Source: CAD feature listing. Evaluate the final solid. Frame: model axes, mm. A direction names the side the tool comes from. Give positions to 0.01 mm unless a question says otherwise; leave off trailing zeros. Order: outer loops, then holes, each group sorted by start corner. A loop starts at its lowest first (then second) coordinate and runs counter-clockwise, first axis right, second up. Notation, with made-up numbers: (85.5, 23.25) - (142.5, 23.25) arc R23 cw to (142.5, 56.25) - close; hole circle Ø5 at (79, 28.5). An arc over 180 degrees is marked (long way). Use CSV: the item, a comma, the result in double quotes.
```python
from build123d import *

# Parameters (mm, degrees)
SKETCH1_W                       = 88.9
SKETCH1_H                       = 107.95
EXTRUDE1_DEPTH                  = 75
SKETCH2_R                       = 14.2875
EXTRUDE2_DEPTH                  = 203.2
M6_TAPPED_HOLE1_D               = 5
M6_TAPPED_HOLE1_DEPTH           = 27.9908
M6_TAPPED_HOLE1_TIP             = 1.502151548
SKETCH6_R                       = 15.875
EXTRUDE4_DEPTH                  = 38.354
SKETCH7_W                       = 88.9
SKETCH7_H                       = 44.45
EXTRUDE5_DEPTH                  = 25
SKETCH8_W                       = 4.2125
SKETCH8_H                       = 107.95
EXTRUDE6_DEPTH                  = 103.538300771
CBORE_FOR_M20_SHCS1_D           = 22
CBORE_FOR_M20_SHCS1_CBORE_D     = 33
CBORE_FOR_M20_SHCS1_CBORE_DEPTH = 20
CHAMFER1_SIZE                   = 1


with BuildPart() as part:
    # Sketch1 → Extrude1 (new body)
    with BuildSketch(Plane(origin=(0, 0, 0), x_dir=(1, 0, 0), z_dir=(0, 1, 0))):
        Rectangle(SKETCH1_W, SKETCH1_H)
    extrude(amount=EXTRUDE1_DEPTH)

    # Sketch2 → Extrude2 (cut)
    with BuildSketch(Plane(origin=(0, 75, 0), x_dir=(1, 0, 0), z_dir=(0, 1, 0))):
        with Locations(Location((-4.7625, 0, 0), (0, 0, 270))):
            Circle(SKETCH2_R)
    extrude(amount=-EXTRUDE2_DEPTH, mode=Mode.SUBTRACT)

    # M6 Tapped Hole1
    with Locations(Plane.XZ):
        with Locations((-22.9235, 34.925), (13.3985, 34.925), (-22.9235, -34.925), (13.3985, -34.925)):
            Hole(M6_TAPPED_HOLE1_D / 2, depth=M6_TAPPED_HOLE1_DEPTH)
            with Locations((0, 0, -(M6_TAPPED_HOLE1_DEPTH + M6_TAPPED_HOLE1_TIP / 2))):  # 118° drill point
                Cone(0, M6_TAPPED_HOLE1_D / 2, M6_TAPPED_HOLE1_TIP, mode=Mode.SUBTRACT)

    # Sketch6 → Extrude4 (cut)
    with BuildSketch(Plane(origin=(0, 75, 0), x_dir=(1, 0, 0), z_dir=(0, 1, 0))):
        with Locations(Location((-4.7625, 0, 0), (0, 0, 270))):
            Circle(SKETCH6_R)
    extrude(amount=-EXTRUDE4_DEPTH, mode=Mode.SUBTRACT)

    # Sketch7 → Extrude5 (cut)
    with BuildSketch(Plane.XZ):
        Rectangle(SKETCH7_W, SKETCH7_H)
    extrude(amount=-EXTRUDE5_DEPTH, mode=Mode.SUBTRACT)

    # Sketch8 → Extrude6 (cut, through all)
    with BuildSketch(Plane(origin=(0, 75, 0), x_dir=(1, 0, 0), z_dir=(0, 1, 0))):
        with Locations((42.34375, 0)):
            Rectangle(SKETCH8_W, SKETCH8_H)
    extrude(amount=-EXTRUDE6_DEPTH, mode=Mode.SUBTRACT)

    # CBORE for M20 SHCS1 (through all)
    with Locations(Plane.ZY.offset(44.45)):
        with Locations((32.5, 50), (-32.5, 50)):
            CounterBoreHole(CBORE_FOR_M20_SHCS1_D / 2, CBORE_FOR_M20_SHCS1_CBORE_D / 2, CBORE_FOR_M20_SHCS1_CBORE_DEPTH)

    # Chamfer1
    chamfer1_edges = [part.edges().sort_by_distance(p)[0] for p in [
        (-4.7625, 75, -15.875),
    ]]
    chamfer(chamfer1_edges, length=CHAMFER1_SIZE)


solid = part.part
```
Item 1: Mould query, pull axis Z, two halves, no side actions, for faces 6 (the flat face through (-3, 37, -53.975)), 7 (the cylindrical face through (-25.233, 14.191, 33.967)), 8 (the flat face through (-3, 0, 38)). Classes: released by +Z, released by -Z, zero draft, split by the parting line, or undercut.
Filled in:
face 6,"released by -Z"
face 7,"undercut"
face 8,"zero draft"
Item 2: Material intervals for line 1 (Y direction, x = -30.5, z = 32.5); line 2 (Z direction, x = 10.5, y = 3) (3 decimals); line 3 (Z direction, x = -24.5, y = 36) (3 decimals), sorted ascending. Write a range as from..to.
Filled in:
line 1,"y = 0..33.5, 66.5..75"
line 2,"z = -53.975..-22.225, 22.225..53.975"
line 3,"z = -53.975..-41.232, -23.768..23.768, 41.232..53.975"
Item 3: Set-up query: faces 1 (the cylindrical face through (-34.59, 33.892, -36.077)), 2 (the flat face through (-44.45, 37, 1)), 3 (the flat face through (-3, 12, -22.225)), 4 (the cylindrical face through (-24.27, 14.19, -32.82)), 5 (the cylindrical face through (10.977, 55.584, -2.067)). Return all of +Z, -Z, +X, -X, +Y, -Y with unobstructed straight access to the full face (end or side cutting, diameter ignored); none if empty.
Filled in:
face 1,"-X"
face 2,"+Z, -Z, -X, +Y, -Y"
face 3,"+X, -X, -Y"
face 4,"-Y"
face 5,"+Y"
Item 4: First-contact query: pin 1 (16.5 mm diameter, centred on y = 49.5, z = -32.5, fed in from -X); pin 2 (2 mm diameter, centred on x = 25.5, z = -6.5, fed in from -Y); pin 3 (4.5 mm diameter, centred on x = -22.92, z = -34.92, fed in from -Y); pin 4 (4 mm diameter, centred on y = 60.5, z = 34, fed in from -X). Flat tips, straight axial feed; report the tip coordinate or a pass-through.
Filled in:
pin 1,"passes through"
pin 2,"stops at y = 25"
pin 3,"stops at y = 28.14"
pin 4,"stops at x = -24.45"
Item 5: Section C-C on x = -28.5. Return the cut outline in (y, z) (3 decimals), then the cut area to 3 significant figures.
Filled in:
outline,"(0, -53.975) - (75, -53.975) - (75, 53.975) - (0, 53.975) - (0, 22.225) - (25, 22.225) - (25, -22.225) - (0, -22.225) - close; hole circle Ø33 at (50, -32.5); hole circle Ø33 at (50, 32.5)"
area,"5,270 mm2"
Item 6: Section B-B on y = 50. Count the separate pieces of the cut face and the enclosed holes in it, then the cut area to 3 significant figures.
Filled in:
separate pieces,"3"
enclosed holes,"1"
area,"4,180 mm2"
